Geometry check sheet. Reference: the model listing, model coordinates, mm. Face numbers are marked on the shaded views. A direction names the side the tool comes from. Coordinates: 2 decimals unless noted, no trailing zeros. Order: outer loops, then holes, each group sorted by start corner. A loop starts at its lowest first (then second) coordinate and runs counter-clockwise, first axis right, second up. Notation, with made-up numbers: M -2.5,-13.75 L 29.5,-13.75 A25 cw 29.5,22.25 Z; hole C -29.75,72.5 d3. An arc over 180 degrees is marked long. One line per item, written item: value. Start each with the question number.
1) Sectioned sample at A-A, the plane x = -2. Enter the section's corners in (y, z) (3 decimals), then the cut area to 3 significant figures.
2) Draft check along Y on the marked faces 3, 4, 5 and 6. Enter one of: pulls with the +Y half, pulls with the -Y half, needs draft (parallel to the pull), parting line crosses it, or undercut.
3) Thickness scan on L1, parallel to Y at x = -7.5, z = 3 (3 decimals); L2, parallel to X at y = 25.5, z = 7.75; L3, parallel to Z at x = 15, y = 37. Record the ranges inside material, lowest first. Write a range as from..to.
4) Sectioned sample at D-D, the plane z = 21. State how many separate pieces and enclosed holes the cut face has, then the cut area to 3 significant figures.
5) Sectioned sample at C-C, the plane y = -49. Enter the section's corners in (x, z), then the cut area to 3 significant figures.
6) Go/stop test with flat-tipped pins: P1, Ø2, axis at x = 2, y = 70.5, coming from the +Z side; P2, Ø6, axis at y = -40.5, z = 12, coming from the +X side; P3, Ø3, axis at x = -0.5, y = -42, coming from the +Z side. Record where each tip stops, or that it passes through.
7) Sectioned sample at B-B, the plane z = 6.25. Enter the section's corners in (x, y) (3 decimals), then the cut area to 3 significant figures.
8) Access from +Z, -Z, +X, -X, +Y, -Y to the whole of each face (thin tool, end or side, straight path). Record for the marked faces 1 and 2.
```python
from build123d import *

# Parameters (mm, degrees)
F0_W     = 71.12
F0_H     = 143.51
F1_DEPTH = 22.86
F2_W     = 66.04
F2_H     = 138.43
F3_DEPTH = 20.32
F5_DEPTH = 71.121
F6_W     = 15.24
F6_H     = 20.32
F7_DEPTH = 25.4


with BuildPart() as f1:
    # F0 (on Top) → F1 (new body)
    with BuildSketch(Plane.XY):
        Rectangle(F0_W, F0_H)
    extrude(amount=F1_DEPTH)

    # F2 (on face) → F3 (cut)
    with BuildSketch(Plane.XY.offset(22.86)):
        Rectangle(F2_W, F2_H)
    extrude(amount=-F3_DEPTH, mode=Mode.SUBTRACT)

    # F4 (on face) → F5 (cut, through all)
    with BuildSketch(Plane.YZ.offset(35.56)):
        with BuildLine():
            Line((-67.944304, 22.86), (-67.944304, 14.064014))
            ThreePointArc((-67.944304, 14.064014), (-61.746635, 7.621811), (-55.248448, 13.760757))
            Line((-55.248448, 13.760757), (-55.248448, 14.179243))
            Line((-55.248448, 14.179243), (-55.248448, 22.86))
            Line((-55.248448, 22.86), (-67.944304, 22.86))
        make_face()
        with BuildLine():
            Line((-55.248448, 14.179243), (-55.248448, 13.760757))
            ThreePointArc((-55.248448, 13.760757), (-55.245, 13.97), (-55.248448, 14.179243))
        make_face()
        with BuildLine():
            Line((-34.928448, 14.179243), (-34.928448, 22.86))
            Line((-34.928448, 22.86), (-47.624304, 22.86))
            Line((-47.624304, 22.86), (-47.624304, 14.064014))
            ThreePointArc((-47.624304, 14.064014), (-41.426635, 7.621811), (-34.928448, 13.760757))
            Line((-34.928448, 13.760757), (-34.928448, 14.179243))
        make_face()
        with BuildLine():
            ThreePointArc((-34.928448, 13.760757), (-34.925, 13.97), (-34.928448, 14.179243))
            Line((-34.928448, 14.179243), (-34.928448, 13.760757))
        make_face()
        with BuildLine():
            Line((-14.608448, 14.179243), (-14.608448, 22.86))
            Line((-14.608448, 22.86), (-27.304304, 22.86))
            Line((-27.304304, 22.86), (-27.304304, 14.064014))
            ThreePointArc((-27.304304, 14.064014), (-21.106635, 7.621811), (-14.608448, 13.760757))
            Line((-14.608448, 13.760757), (-14.608448, 14.179243))
        make_face()
        with BuildLine():
            ThreePointArc((-14.608448, 13.760757), (-14.605, 13.97), (-14.608448, 14.179243))
            Line((-14.608448, 14.179243), (-14.608448, 13.760757))
        make_face()
        with BuildLine():
            Line((5.711552, 14.179243), (5.711552, 22.86))
            Line((5.711552, 22.86), (-6.984304, 22.86))
            Line((-6.984304, 22.86), (-6.984304, 14.064014))
            ThreePointArc((-6.984304, 14.064014), (-0.786635, 7.621811), (5.711552, 13.760757))
            Line((5.711552, 13.760757), (5.711552, 14.179243))
        make_face()
        with BuildLine():
            ThreePointArc((5.711552, 13.760757), (5.715, 13.97), (5.711552, 14.179243))
            Line((5.711552, 14.179243), (5.711552, 13.760757))
        make_face()
        with BuildLine():
            Line((26.031552, 14.179243), (26.031552, 22.86))
            Line((26.031552, 22.86), (13.335696, 22.86))
            Line((13.335696, 22.86), (13.335696, 14.064014))
            ThreePointArc((13.335696, 14.064014), (19.533365, 7.621811), (26.031552, 13.760757))
            Line((26.031552, 13.760757), (26.031552, 14.179243))
        make_face()
        with BuildLine():
            ThreePointArc((26.031552, 13.760757), (26.035, 13.97), (26.031552, 14.179243))
            Line((26.031552, 14.179243), (26.031552, 13.760757))
        make_face()
        with BuildLine():
            Line((52.705696, 22.86), (52.705696, 14.064014))
            ThreePointArc((52.705696, 14.064014), (58.903365, 7.621811), (65.401552, 13.760757))
            Line((65.401552, 13.760757), (65.401552, 14.179243))
            Line((65.401552, 14.179243), (65.401552, 22.86))
            Line((65.401552, 22.86), (52.705696, 22.86))
        make_face()
        with BuildLine():
            Line((65.401552, 14.179243), (65.401552, 13.760757))
            ThreePointArc((65.401552, 13.760757), (65.405, 13.97), (65.401552, 14.179243))
        make_face()
    extrude(amount=-F5_DEPTH, mode=Mode.SUBTRACT)

    # F6 (on face) → F7 (cut)
    with BuildSketch(Plane(origin=(0, 71.755, 0), x_dir=(-1, 0, 0), z_dir=(0, 1, 0))):
        with Locations((0, 22.86)):
            Rectangle(F6_W, F6_H)
    extrude(amount=-F7_DEPTH, mode=Mode.SUBTRACT)


solid = f1.part
```
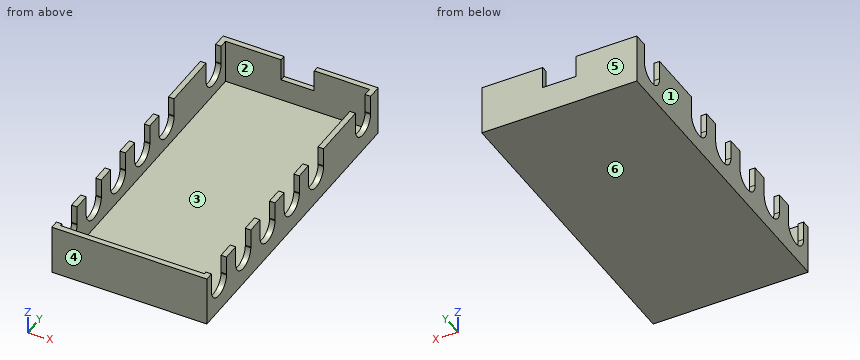
Final values:
1. outline: M -71.755,0 L 71.755,0 L 71.755,12.7 L 69.215,12.7 L 69.215,2.54 L -69.215,2.54 L -69.215,22.86 L -71.755,22.86 Z
1. area: 442 mm^2
2. face 3: undercut
2. face 4: pulls with the -Y half
2. face 5: pulls with the +Y half
2. face 6: needs draft
3. L1: y = -71.755..-69.215, 69.215..71.755
3. L2: x = -35.56..-33.02, 33.02..35.56
3. L3: z = 0..2.54
4. separate pieces: 13
4. enclosed holes: 0
4. area: 639 mm^2
5. outline: M -35.56,0 L 35.56,0 L 35.56,22.86 L 33.02,22.86 L 33.02,2.54 L -33.02,2.54 L -33.02,22.86 L -35.56,22.86 Z
5. area: 284 mm^2
6. P1: stops at z = 12.7
6. P2: passes through
6. P3: stops at z = 2.54
7. outline: M -35.56,-71.755 L 35.56,-71.755 L 35.56,71.755 L -35.56,71.755 Z; hole M -33.02,-69.215 L 33.02,-69.215 L 33.02,69.215 L -33.02,69.215 Z
7. area: 1,060 mm^2
8. face 1: +Z, -Z, -X, +Y, -Y
8. face 2: +Z
